Check sheet for the modelled part. Datum: model origin and axes. Units: mm. A direction names the side the tool comes from. Round coordinates to 2 decimals unless told otherwise and drop trailing zeros. Order: outer loops, then holes, each group sorted by start corner. A loop starts at its lowest first (then second) coordinate and runs counter-clockwise, first axis right, second up. Notation, with made-up numbers: (79, -39.75) -> (123, -39.75) arc R24 ccw to (123, -28.75) -> close; hole circle Ø3 at (-7.75, -15). An arc over 180 degrees is marked (long way). Answer in a Markdown table with one row per item. Add a question column.
1. Sectioned sample at A-A, the plane y = 9. Record the boundary of the cut face in (x, z), then the cut area to 3 significant figures.
2. Depth check by flat-ended pin: P1, Ø11, axis at x = -3, z = -1.5, coming from the -Y side; P2, Ø5, axis at x = 0, z = 0, coming from the +Y side; P3, Ø1, axis at x = 1, y = 6, coming from the +Z side; P4, Ø4, axis at x = 2, y = 29, coming from the +Z side. Enter the tip coordinate at first touch or a pass-through.
3. Sectioned sample at B-B, the plane y = 14. Record the boundary of the cut face in (x, z), then the cut area to 3 significant figures.
4. Material ranges on L1, parallel to Z at x = 0, y = 29.5; L2, parallel to Z at x = 0, y = 6.5; L3, parallel to X at y = 11.25, z = 0, recorded low to high. Write a range as from..to.
5. Access from +Z, -Z, +X, -X, +Y, -Y to the whole of each face (thin tool, end or side, straight path). Record for faces 3 (the cylindrical face through (-1.276, 6.74, -5.745)), 4 (the cylindrical face through (10.635, 20.507, -3.349)).
6. Draft check along Y on faces 1 (the cylindrical face through (-1.73, 28.01, 7.81)), 2 (the flat face through (5, 6, 5)). Enter one of: +Y half, -Y half, draft (parallel to the pull), parting line (faces both ways), or undercut.
Autodesk Inventor part; units mm, degrees
ref_plane "YZ Plane" through (0, 0, 0) normal (1, 0, 0) x (0, 1, 0)
ref_plane "XZ Plane" through (0, 0, 0) normal (0, 1, 0) x (-1, 0, 0)
ref_plane "XY Plane" through (0, 0, 0) normal (0, 0, 1) x (1, 0, 0)
sketch "Sketch1" plane through (0, 0, 0) normal (0, 0, 1) x (1, 0, 0)
  line L0 (0, 0) -> (11.15, 0)
  line L1 (11.15, 0) -> (11.15, 26)
  line L2 (11.15, 26) -> (8, 26)
  line L3 (8, 42.7) -> (0, 42.7)
  line L4 (0, 42.7) -> (0, 0)
  line L5 (8, 39) -> (6, 39)
  line L6 (6, 39) -> (6, 33)
  line L7 (6, 33) -> (8, 33)
  line L8 (8, 26) -> (5, 26)
  line L9 (5, 26) -> (5, 27.5)
  line L10 (5, 27.5) -> (8, 27.5)
  line L11 (8, 28.5) -> (5, 28.5)
  line L12 (5, 28.5) -> (5, 30)
  line L13 (5, 30) -> (8, 30)
  line L14 (8, 39) -> (8, 42.7)
  line L15 (8, 27.5) -> (8, 28.5)
  line L16 (8, 30) -> (8, 33)
  dimension "d7" = 11.15
  dimension "d10" = 8
  dimension "d11" = 42.7
  dimension "d12" = 26
  dimension "d14" = 6
  dimension "d15" = 3.7
  dimension "d16" = 3
  dimension "d17" = 6
  dimension "d18" = 1
  dimension "d19" = 2.5
  dimension "d20" = 5
revolve "Revolution1" add sketch "Sketch1" angle 360 about axis through (0, 42.7, 0) along (0, -1, 0)
sketch "Sketch2" plane through (0, 42.7, 0) normal (0, 1, 0) x (1, 0, 0)
  circle A0 centre (0, 0) radius 8
  circle A1 centre (0, 0) radius 8
hole "Hole1" at (0, 42.7, 0) direction (0, -1, 0) diameter 4.2 end through all
sketch "Sketch3" plane through (0, 42.7, 0) normal (0, 1, 0) x (1, 0, 0)
  circle A0 centre (0, 0) radius 2.1
  circle A1 centre (0, 0) radius 8
hole "Hole2" at (0, 42.7, 0) direction (0, -1, 0) diameter 8 depth 6 tip angle 118
sketch "Sketch4" plane through (0, 0, 0) normal (0, -1, 0) x (1, 0, 0)
  circle A0 centre (0, 0) radius 2.1
  circle A1 centre (0, 0) radius 11.15
hole "Hole3" at (0, 0, 0) direction (0, 1, 0) diameter 5.917 depth 19.1 tip angle 118
sketch "Sketch5" plane through (0, 0, 0) normal (0, 0, 1) x (1, 0, 0)
  line L0 (5, 27.5) -> (5, 26)
  line L1 (-11.15, 26) -> (11.15, 26)
  line L2 (11.15, 26) -> (11.15, 0)
  line L3 (-11.15, 0) -> (11.15, 0)
  line L4 (5, 26) -> (6.15, 0)
  line L5 (11.15, 2.5) -> (6.1058, 2.5)
  line L6 (6.1058, 2.5) -> (6.1058, 1)
  line L7 (6.1058, 1) -> (11.15, 1)
  line L8 (11.15, 1) -> (11.15, 2.5)
  line L9 (11.15, 5) -> (5.9952, 5)
  line L10 (5.9952, 5) -> (5.9952, 3.5)
  line L11 (5.9952, 3.5) -> (11.15, 3.5)
  line L12 (11.15, 3.5) -> (11.15, 5)
  line L13 (11.15, 7.5) -> (5.8846, 7.5)
  line L14 (5.8846, 7.5) -> (5.8846, 6)
  line L15 (5.8846, 6) -> (11.15, 6)
  line L16 (11.15, 6) -> (11.15, 7.5)
  line L17 (11.15, 10) -> (5.774, 10)
  line L18 (5.774, 10) -> (5.774, 8.5)
  line L19 (5.774, 8.5) -> (11.15, 8.5)
  line L20 (11.15, 8.5) -> (11.15, 10)
  line L21 (11.15, 12.5) -> (5.6635, 12.5)
  line L22 (5.6635, 12.5) -> (5.6635, 11)
  line L23 (5.6635, 11) -> (11.15, 11)
  line L24 (11.15, 11) -> (11.15, 12.5)
  line L25 (11.15, 15) -> (5.5529, 15)
  line L26 (5.5529, 15) -> (5.5529, 13.5)
  line L27 (5.5529, 13.5) -> (11.15, 13.5)
  line L28 (11.15, 13.5) -> (11.15, 15)
  line L29 (11.15, 17.5) -> (5.4423, 17.5)
  line L30 (5.4423, 17.5) -> (5.4423, 16)
  line L31 (5.4423, 16) -> (11.15, 16)
  line L32 (11.15, 16) -> (11.15, 17.5)
  line L33 (11.15, 20) -> (5.3317, 20)
  line L34 (5.3317, 20) -> (5.3317, 18.5)
  line L35 (5.3317, 18.5) -> (11.15, 18.5)
  line L36 (11.15, 18.5) -> (11.15, 20)
  line L37 (11.15, 22.5) -> (5.2212, 22.5)
  line L38 (5.2212, 22.5) -> (5.2212, 21)
  line L39 (5.2212, 21) -> (11.15, 21)
  line L40 (11.15, 21) -> (11.15, 22.5)
  line L41 (11.15, 25) -> (5.1106, 25)
  line L42 (5.1106, 25) -> (5.1106, 23.5)
  line L43 (5.1106, 23.5) -> (11.15, 23.5)
  line L44 (11.15, 23.5) -> (11.15, 25)
  line L45 (0, -8.54) -> (0, 51.24)
  point P0 (0, 0)
  dimension "d42" = 1
  dimension "d43" = 2.5
  dimension "d46" = 5
  dimension "d47" = 1
  dimension "d48" = 2.5
  dimension "d49" = 1
  dimension "d50" = 2.5
  dimension "d51" = 1
  dimension "d52" = 2.5
  dimension "d53" = 1
  dimension "d54" = 2.5
  dimension "d55" = 1
  dimension "d56" = 2.5
  dimension "d57" = 1
  dimension "d58" = 2.5
  dimension "d59" = 1
  dimension "d60" = 2.5
  dimension "d61" = 1
  dimension "d62" = 2.5
  dimension "d63" = 1
  dimension "d64" = 2.5
revolve "Revolution2" cut sketch "Sketch5" angle 360 about axis through (0, -10, 0) along (0, 1, 0) contours L42 L41 L2 L43 | L38 L37 L2 L39 | L34 L33 L2 L35 | L6 L5 L2 L7 | L30 L29 L2 L31 | L10 L9 L2 L11 | L26 L25 L2 L27 | L14 L13 L2 L15 | L22 L21 L2 L23 | L18 L17 L2 L19
equation "\"d47\" = d42"
equation "\"d48\" = d43"
equation "\"d49\" = d42"
equation "\"d50\" = d43"
equation "\"d51\" = d42"
equation "\"d52\" = d43"
equation "\"d53\" = d42"
equation "\"d54\" = d43"
equation "\"d55\" = d42"
equation "\"d56\" = d43"
equation "\"d57\" = d42"
equation "\"d58\" = d43"
equation "\"d59\" = d42"
equation "\"d60\" = d43"
equation "\"d61\" = d42"
equation "\"d62\" = d43"
equation "\"d63\" = d42"
equation "\"d64\" = d43"
properties part number "Heatsink" material "Aluminum 6061"
Answer key:
| question | item | result |
|---|---|---|
| 1 | outline | circle Ø11.55 at (0, 0); hole circle Ø5.92 at (0, 0) |
| 1 | area | 77.2 mm² |
| 2 | P1 | stops at y = 0 |
| 2 | P2 | stops at y = 35.8 |
| 2 | P3 | stops at z = 11.14 |
| 2 | P4 | stops at z = 8 |
| 3 | outline | circle Ø11.11 at (0, 0); hole circle Ø5.92 at (0, 0) |
| 3 | area | 69.4 mm² |
| 4 | L1 | z = -5..-2.1, 2.1..5 |
| 4 | L2 | z = -5.88..-2.96, 2.96..5.88 |
| 4 | L3 | x = -5.66..-2.96, 2.96..5.66 |
| 5 | face 3 | none |
| 5 | face 4 | +Y, -Y |
| 6 | face 1 | draft |
| 6 | face 2 | undercut |
